from build123d import *

# Parameters (mm, degrees)
ESQUISSE1_R                     = 2
BOSS_EXTRU_1_DEPTH              = 218
CONG_1_R                        = 0.75
DIAM_TRE_DU_PER_AGE_12_0_12_2_D = 12


with BuildPart() as part:
    # Esquisse1 → Boss.-Extru.1 (new, symmetric)
    with BuildSketch(Plane(origin=(0, 0, 0), x_dir=(0, 0, -1), z_dir=(1, 0, 0))):
        Polygon((2.5, 10), (10, 10), (10, 2.5), (8.5, 2.5), (8.5, 7.439339828), (3.75, 2.689339828), (3.75, -2.689339828), (8.5, -7.439339828), (8.5, -2.5), (10, -2.5), (10, -10), (2.5, -10), (2.5, -8.5), (7.439339828, -8.5), (2.689339828, -3.75), (-2.689339828, -3.75), (-7.439339828, -8.5), (-2.5, -8.5), (-2.5, -10), (-10, -10), (-10, -2.5), (-8.5, -2.5), (-8.5, -7.439339828), (-3.75, -2.689339828), (-3.75, 2.689339828), (-8.5, 7.439339828), (-8.5, 2.5), (-10, 2.5), (-10, 10), (-2.5, 10), (-2.5, 8.5), (-7.439339828, 8.5), (-2.689339828, 3.75), (2.689339828, 3.75), (7.439339828, 8.5), (2.5, 8.5), align=None)
        Circle(ESQUISSE1_R, mode=Mode.SUBTRACT)
    extrude(amount=BOSS_EXTRU_1_DEPTH, both=True)

    # Congé1
    cong_1_edges = [part.edges().sort_by_distance(p)[0] for p in [
        (0, 7.439339828, -8.5),
        (0, -7.439339828, -8.5),
        (0, -8.5, -7.439339828),
        (0, -8.5, 7.439339828),
        (0, -7.439339828, 8.5),
        (0, 7.439339828, 8.5),
        (0, 8.5, 7.439339828),
        (0, 8.5, -7.439339828),
    ]]
    fillet(cong_1_edges, radius=CONG_1_R)

    # Diamètre du perçage Ø12.0 (12)2 (through all)
    with Locations(Plane(origin=(0, 10, 0), x_dir=(1, 0, 0), z_dir=(0, 1, 0))):
        with Locations((0, 0)):
            Hole(DIAM_TRE_DU_PER_AGE_12_0_12_2_D / 2)


solid = part.part
Source: CAD feature listing. Evaluate the final solid. Frame: model axes, mm. Round coordinates to 2 decimals unless told otherwise and drop trailing zeros. One line per item, written item: value. Start each with the question number.
Item 1: Ray query, L1, parallel to Z at x = -163.5, y = 5.25; L2, parallel to Y at x = 128, z = 0.5; L3, parallel to Z at x = 93.5, y = 0. Return the intervals inside material, ascending. Write a range as from..to.
Item 2: Pin query (flat end, axial travel): pin 1 (1.5 mm diameter, centred on x = 41.5, y = 1, fed in from +Z). Return the tip coordinate at first contact, or that it passes through.
Item 3: Mould query, pull axis Z, two halves, no side actions, for faces 1 (the flat face through (3, 10, 6)), 2 (the cylindrical face through (-5.54, -0.11, 2.3)), 3 (the flat face through (3, -6, 10)). Classes: pulls with the +Z half, pulls with the -Z half, needs draft (parallel to the pull), parting line crosses it, or undercut.
Result set:
1. L1: z = -10..-8.5, -6.31..-4.19, 4.19..6.31, 8.5..10
1. L2: y = -3.75..-1.94, 1.94..3.75
1. L3: z = -3.75..-2, 2..3.75
2. pin 1: stops at z = 3.75
3. face 1: needs draft
3. face 2: undercut
3. face 3: pulls with the +Z half
